```python
from build123d import *

# Parameters (mm, degrees)
SKETCH1_W                       = 40
SKETCH1_H                       = 25
BOSS_EXTRUDE1_DEPTH             = 10
BOSS_EXTRUDE2_DEPTH             = 10
EXTRUDE_THIN1_DEPTH             = 30
EXTRUDE_THIN1_DEPTH_BACK        = 10
FILLET1_R                       = 8
SKETCH4_R                       = 8
SKETCH4_W                       = 11
SKETCH4_H                       = 5
SKETCH4_H_2                     = 4
CUT_EXTRUDE1_DEPTH              = 30
CIRPATTERN1_COUNT               = 2
CIRPATTERN1_ANGLE               = 28
CIRPATTERN1_THE_OTHER_WAY_COUNT = 2
CIRPATTERN1_THE_OTHER_WAY_ANGLE = 28
BOSS_EXTRUDE3_DEPTH             = 25
SKETCH7_R                       = 2
CUT_EXTRUDE2_DEPTH              = 11


with BuildPart() as part:
    # Sketch1 → Boss-Extrude1 (new body)
    with BuildSketch(Plane(origin=(0, 0, 0), x_dir=(1, 0, 0), z_dir=(0, 1, 0))):
        with Locations((20, 12.5)):
            Rectangle(SKETCH1_W, SKETCH1_H)
    extrude(amount=BOSS_EXTRUDE1_DEPTH)

    # Sketch2 → Boss-Extrude2 (add)
    with BuildSketch(Plane(origin=(0, 10, 0), x_dir=(1, 0, 0), z_dir=(0, 1, 0))):
        Polygon((43, -40), (-3, -40), (-43.615589272, -18.404308112), (-43.615589272, 0), (0, 0), (40, 0), (83.615589272, 0), (83.615589272, -18.404308112), align=None)
    extrude(amount=-BOSS_EXTRUDE2_DEPTH)

    # Sketch3 → Extrude-Thin1 (add, two sides)
    with BuildSketch(Plane(origin=(0, 10, 0), x_dir=(1, 0, 0), z_dir=(0, 1, 0))) as extrude_thin1_sk:
        Polygon((-43.615589272, 0), (-43.615589272, -18.404308112), (-3, -40), (43, -40), (83.615589272, -18.404308112), (83.615589272, 0), (95.615589272, 0), (95.615589272, -25.61463554), (45.991936034, -52), (-5.991936034, -52), (-55.615589272, -25.61463554), (-55.615589272, 0), align=None)
    extrude(amount=EXTRUDE_THIN1_DEPTH)
    extrude(extrude_thin1_sk.sketch, amount=-EXTRUDE_THIN1_DEPTH_BACK)

    # Fillet1
    fillet1_edges = [part.edges().sort_by_distance(p)[0] for p in [
        (95.615589272, 20, 25.61463554),
        (45.991936034, 20, 52),
        (-5.991936034, 20, 52),
        (-55.615589272, 20, 25.61463554),
    ]]
    fillet(fillet1_edges, radius=FILLET1_R)

    # Sketch4 → Cut-Extrude1 (cut)
    with BuildSketch(Plane(origin=(0, 0, 40), x_dir=(-1, 0, 0), z_dir=(0, 0, -1))):
        with Locations((-32.8, 25)):
            Circle(SKETCH4_R)
        with Locations((-7.2, 25)):
            Circle(SKETCH4_R)
        with Locations((-20, 17.2)):
            Rectangle(SKETCH4_W, SKETCH4_H)
        with Locations((-20, 33.3)):
            Rectangle(SKETCH4_W, SKETCH4_H_2)
    cut_extrude1 = extrude(amount=-CUT_EXTRUDE1_DEPTH, mode=Mode.SUBTRACT)

    # CirPattern1: Cut-Extrude1 ×2 about axis
    cirpattern1_axis = Axis((20, 40, -52.247961471), (0, 1, 0))
    for i in range(1, CIRPATTERN1_COUNT):
        add(cut_extrude1.rotate(cirpattern1_axis, i * CIRPATTERN1_ANGLE / (CIRPATTERN1_COUNT - 1)), mode=Mode.SUBTRACT)

    # CirPattern1 the other way: Cut-Extrude1 ×2 about axis
    cirpattern1_the_other_way_axis = Axis((20, 40, -52.247961471), (0, -1, 0))
    for i in range(1, CIRPATTERN1_THE_OTHER_WAY_COUNT):
        add(cut_extrude1.rotate(cirpattern1_the_other_way_axis, i * CIRPATTERN1_THE_OTHER_WAY_ANGLE / (CIRPATTERN1_THE_OTHER_WAY_COUNT - 1)), mode=Mode.SUBTRACT)

    # Sketch6 → Boss-Extrude3 (add)
    with BuildSketch(Plane(origin=(0, 40, 0), x_dir=(1, 0, 0), z_dir=(0, 1, 0))):
        with BuildLine():
            Line((47.753084514, -51.063580743), (91.371361774, -27.871331331))
            ThreePointArc((91.371361774, -27.871331331), (94.472927677, -24.928055187), (95.615589272, -20.807750588))
            Line((95.615589272, -20.807750588), (95.615589272, 0))
            Line((95.615589272, 0), (83.615589272, 0))
            Line((83.615589272, 0), (83.615589272, -18.404308112))
            Line((83.615589272, -18.404308112), (43, -40))
            Line((43, -40), (-3, -40))
            Line((-3, -40), (-43.615589272, -18.404308112))
            Line((-43.615589272, -18.404308112), (-43.615589272, 0))
            Line((-43.615589272, 0), (-55.615589272, 0))
            Line((-55.615589272, 0), (-55.615589272, -20.807750588))
            ThreePointArc((-55.615589272, -20.807750588), (-54.472927677, -24.928055187), (-51.371361774, -27.871331331))
            Line((-51.371361774, -27.871331331), (-7.753084514, -51.063580743))
            ThreePointArc((-7.753084514, -51.063580743), (-5.932687176, -51.76236581), (-3.997312011, -52))
            Line((-3.997312011, -52), (43.997312011, -52))
            ThreePointArc((43.997312011, -52), (45.932687176, -51.76236581), (47.753084514, -51.063580743))
        make_face()
    extrude(amount=BOSS_EXTRUDE3_DEPTH)

    # Sketch7 → Cut-Extrude2 (cut, through all)
    with BuildSketch(Plane(origin=(0, 10, 0), x_dir=(1, 0, 0), z_dir=(0, 1, 0))):
        with Locations((10, 12.5)):
            Circle(SKETCH7_R)
        with Locations((30, 12.5)):
            Circle(SKETCH7_R)
    extrude(amount=-CUT_EXTRUDE2_DEPTH, mode=Mode.SUBTRACT)


solid = part.part
```
Check sheet for the modelled part. Datum: model origin and axes. Units: mm. A direction names the side the tool comes from. Coordinates: 2 decimals unless noted, no trailing zeros. Write each loop counter-clockwise with the first axis right and the second up, starting at its lowest first coordinate (ties: lowest second). Pieces come first, ordered by that corner, then holes. Notation, with made-up numbers: (23, 75.5) -> (65, 75.5) arc R21 ccw to (65, 79.5) -> close; hole circle Ø5 at (5, 66). An arc over 180 degrees is marked (long way). Use a Markdown table: item, result.
1. Sectioned sample at B-B (x = 10). Enter the section's corners in (y, z), plus the area to 3 significant figures.
Reported:
| item | result |
|---|---|
| outline | (0, -25) -> (10, -25) -> (10, -14.5) -> (0, -14.5) -> close; (0, -10.5) -> (10, -10.5) -> (10, 40) -> (17.51, 40) -> (17.51, 52) -> (0, 52) -> close; (32.49, 40) -> (65, 40) -> (65, 52) -> (32.49, 52) -> close |
| area | 1,210 mm2 |
2. Sectioned sample at A-A (y = 7). Enter the section's corners in (x, z), plus the area to 3 significant figures.
Reported:
| item | result |
|---|---|
| outline | (-55.62, 0) -> (0, 0) -> (0, -25) -> (40, -25) -> (40, 0) -> (95.62, 0) -> (95.62, 20.81) arc R8 ccw to (91.37, 27.87) -> (47.75, 51.06) arc R8 ccw to (44, 52) -> (-4, 52) arc R8 ccw to (-7.75, 51.06) -> (-51.37, 27.87) arc R8 ccw to (-55.62, 20.81) -> close; hole circle Ø4 at (10, -12.5); hole circle Ø4 at (30, -12.5) |
| area | 7,520 mm2 |
3. Scan lines: line 1 along Y through (x, z) = (24, 46); line 2 along X through (y, z) = (6.25, -12.5); line 3 along X through (y, z) = (28, 2.5). Record each from-to range of solid material in increasing order.
Reported:
| item | result |
|---|---|
| line 1 | y = 0 to 14.7, 19.7 to 31.3, 35.3 to 65 |
| line 2 | x = 0 to 8, 12 to 28, 32 to 40 |
| line 3 | x = -55.62 to -43.62, 83.62 to 95.62 |
4. Go/stop test with flat-tipped pins: pin 1 Ø3 at (y, z) = (34, 44) entering from +X; pin 2 Ø8 at (x, y) = (28, 36) entering from -Z; pin 3 Ø2 at (y, z) = (33, 46.5) entering from -X. Record where each tip stops, or that it passes through.
Reported:
| item | result |
|---|---|
| pin 1 | stops at x = 63.86 |
| pin 2 | stops at z = 40 |
| pin 3 | stops at x = -18.22 |
5. Release check for a two-part mould opening along Y. For faces 5 (the flat face through (66, 14.7, 34)), 6 (the flat face through (-43.616, 37, 9)) record: pulls with the +Y half, pulls with the -Y half, needs draft (parallel to the pull), parting line crosses it, or undercut.
Reported:
| item | result |
|---|---|
| face 5 | undercut |
| face 6 | needs draft |
6. Sectioned sample at D-D (z = 44). Give the number of separate pieces and of enclosed holes in the cut face, plus the area to 3 significant figures.
Reported:
| item | result |
|---|---|
| separate pieces | 1 |
| enclosed holes | 4 |
| area | 4,470 mm2 |
7. Sectioned sample at C-C (y = 37). Enter the section's corners in (x, z), plus the area to 3 significant figures.
Reported:
| item | result |
|---|---|
| outline | (-55.62, 0) -> (-43.62, 0) -> (-43.62, 18.4) -> (-3, 40) -> (43, 40) -> (83.62, 18.4) -> (83.62, 0) -> (95.62, 0) -> (95.62, 20.81) arc R8 ccw to (91.37, 27.87) -> (47.75, 51.06) arc R8 ccw to (44, 52) -> (-4, 52) arc R8 ccw to (-7.75, 51.06) -> (-51.37, 27.87) arc R8 ccw to (-55.62, 20.81) -> close |
| area | 2,330 mm2 |
8. Tool access check on faces 1 (the flat face through (-30.94, 33.27, 31.84)), 2 (the flat face through (-26, 35.3, 34)), 3 (the flat face through (-23.023, 43.226, 29.353)), 4 (the flat face through (20, 19.7, 46)). Record the directions out of +Z, -Z, +X, -X, +Y, -Y that give a thin tool (end or side, any length) a straight path to the whole face; none if there is none.
Reported:
| item | result |
|---|---|
| face 1 | +Z |
| face 2 | none |
| face 3 | -Z, +Y |
| face 4 | +Z, -Z |
